Here's the drawing with two shaded views (mm, measured from the low corner). I have some questions. A direction names the side the tool comes from. Give positions to 0.01 mm unless a question says otherwise; leave off trailing zeros. Write each loop counter-clockwise with the first axis right and the second up, starting at its lowest first coordinate (ties: lowest second). Pieces come first, ordered by that corner, then holes. Notation, with made-up numbers: (30.25, 50.5) - (56.25, 50.5) arc R5 ccw to (56.25, 58.5) - close; hole circle Ø4 at (15, 19.5). An arc over 180 degrees is marked (long way). Write item = value, one per line.
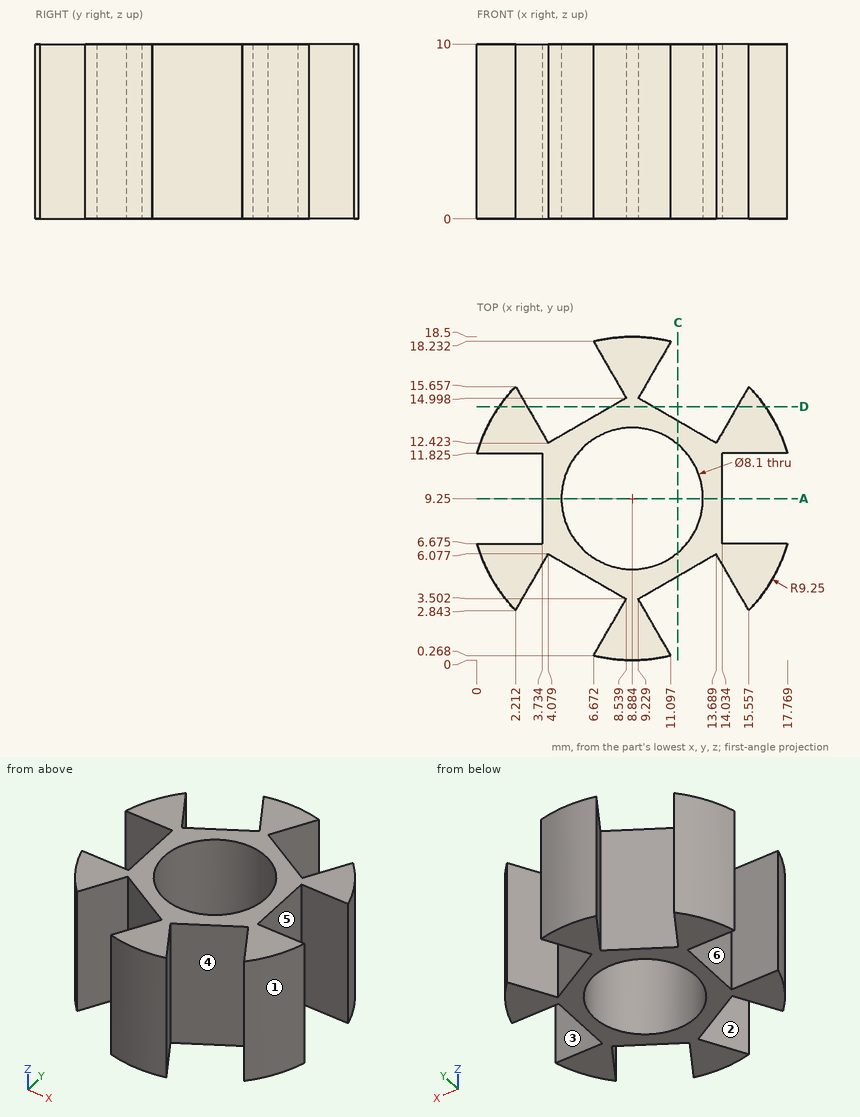
1. Which directions (+Z, -Z, +X, -X, +Y, -Y) give clear straight access to the entire face, cutting with the end or side of a thin tool? Please do the marked faces 4, 5 and 6.
Filled sheet:
face_4 = +Z, -Z
face_5 = +Z, -Z, +X
face_6 = +Z, -Z, -X
2. Thinking about a two-plate mould opening in X: for the marked faces 1, 2 and 3, which applies, pulls with the +X half, pulls with the -X half, needs draft (parallel to the pull), parting line crosses it, or undercut?
Filled sheet:
face_1 = pulls with the +X half
face_2 = undercut
face_3 = needs draft
3. I need wall thicknesses on line 1 (Y direction, x = 10.75, z = 7) (1 decimal); line 2 (X direction, y = 13.5, z = 3) (1 decimal); line 3 (Y direction, x = 15.5, z = 6) (1 decimal). Which ranges of each line are inside material? Lowest first, please.
Filled sheet:
line_1 = 0.2 to 0.9, 4.4 to 5.7, 12.8 to 14.1, 17.6 to 18.3
line_2 = 0.7 to 3.5, 5.9 to 11.8, 14.3 to 17.1
line_3 = 2.9 to 6.7, 11.8 to 15.6
4. If we section it at D-D, the plane y = 14.5: Please give me the cut outline in (x, z).
Filled sheet:
outline = (1.27, 0) - (2.88, 0) - (2.88, 10) - (1.27, 10) - close; (7.68, 0) - (10.09, 0) - (10.09, 10) - (7.68, 10) - close; (14.89, 0) - (16.5, 0) - (16.5, 10) - (14.89, 10) - close
5. For pin 1 (8 mm diameter, centred on x = 10.5, y = 16.5, fed in from +Z); pin 2 (2.5 mm diameter, centred on y = 10.5, z = 5, fed in from +X); pin 3 (4 mm diameter, centred on x = 15.5, z = 3.5, fed in from -Y); pin 4 (1.5 mm diameter, centred on x = 7.5, y = 10, fed in from -Z), each with a flat end and sliding along its axis, tell me the tip position at first contact or that it passes through.
Filled sheet:
pin_1 = 10
pin_2 = 14.03
pin_3 = 2.84
pin_4 = through
6. If we section it at A-A, the plane y = 9.25: Please give me the cut outline in (x, z) (1 decimal).
Filled sheet:
outline = (3.7, 0) - (4.8, 0) - (4.8, 10) - (3.7, 10) - close; (12.9, 0) - (14, 0) - (14, 10) - (12.9, 10) - close
7. If we section it at C-C, the plane x = 11.5: Please give me the cut outline in (y, z).
Filled sheet:
outline = (4.81, 0) - (6.16, 0) - (6.16, 10) - (4.81, 10) - close; (12.34, 0) - (13.69, 0) - (13.69, 10) - (12.34, 10) - close
